```python
from build123d import *

# Parameters (mm, degrees)
SKETCH1_W           = 25.4
SKETCH1_H           = 25.4
BOSS_EXTRUDE1_DEPTH = 38.1
CUT_EXTRUDE1_DEPTH  = 43.121134838
CUT_EXTRUDE2_START  = -3.175
CUT_EXTRUDE2_DEPTH  = 31.75
SKETCH4_R           = 3.175
CUT_EXTRUDE3_DEPTH  = 48.519048812
SKETCH5_R           = 3.175
CUT_EXTRUDE5_DEPTH  = 48.519048812


with BuildPart() as part:
    # Sketch1 → Boss-Extrude1 (new body)
    with BuildSketch(Plane(origin=(0, 0, 0), x_dir=(1, 0, 0), z_dir=(0, 1, 0))):
        Rectangle(SKETCH1_W, SKETCH1_H)
    extrude(amount=BOSS_EXTRUDE1_DEPTH)

    # Sketch2 → Cut-Extrude1 (cut, through all)
    with BuildSketch(Plane(origin=(0, 38.1, 0), x_dir=(1, 0, 0), z_dir=(0, 1, 0))):
        Polygon((-12.7, 12.7), (12.7, -12.7), (-12.7, -12.7), align=None)
    extrude(amount=-CUT_EXTRUDE1_DEPTH, mode=Mode.SUBTRACT)

    # Sketch3 → Cut-Extrude2 (cut)
    with BuildSketch(Plane(origin=(0, 38.1, 0), x_dir=(1, 0, 0), z_dir=(0, 1, 0)).offset(CUT_EXTRUDE2_START)):
        Polygon((-9.525, 9.525), (9.525, 9.525), (9.525, -9.525), align=None)
    extrude(amount=-CUT_EXTRUDE2_DEPTH, mode=Mode.SUBTRACT)

    # Sketch4 → Cut-Extrude3 (cut, through all)
    with BuildSketch(Plane(origin=(0, 0, -12.7), x_dir=(-1, 0, 0), z_dir=(0, 0, -1))):
        with Locations((0, 19.05)):
            Circle(SKETCH4_R)
    extrude(amount=-CUT_EXTRUDE3_DEPTH, mode=Mode.SUBTRACT)

    # Sketch5 → Cut-Extrude5 (cut, through all)
    with BuildSketch(Plane(origin=(12.7, 0, 0), x_dir=(0, 0, -1), z_dir=(1, 0, 0))):
        with Locations((0, 31.75)):
            Circle(SKETCH5_R)
        with Locations((0, 6.35)):
            Circle(SKETCH5_R)
    extrude(amount=-CUT_EXTRUDE5_DEPTH, mode=Mode.SUBTRACT)


solid = part.part
```
CAD build for the part. Positions are in the model's coordinates, mm. A direction names the side the tool comes from. Coordinates: 2 decimals unless noted, no trailing zeros. Loops run counter-clockwise (first coordinate to the right, second up) from the corner with the lowest first, then second, coordinate; pieces in that order, holes last. Notation, with made-up numbers: (88, 57.5) - (101, 57.5) arc R22 ccw to (101, 79.5) - close; hole circle Ø7 at (35.5, 32.25). An arc over 180 degrees is marked (long way). Use CSV: the item, a comma, the result in double quotes. Start each with the question number.
Q1. Cut at C-C, the plane x = 5.25. List the corners of the cut face in (y, z) (3 decimals).
Q2. Cut at D-D, the plane y = 6.35. List the corners of the cut face in (x, z) (3 decimals), then the cut area to 3 significant figures.
Q3. Two-plate mould, pull along Y, no slides. Class faces 3 (the cylindrical face through (0.69, 15.95, -11.13)), 4 (the flat face through (5, 38.1, -6)), 5 (the flat face through (5, 0, -6)), 6 (the flat face through (0, 23, -12.7)): +Y half, -Y half, draft (parallel to the pull), parting line (faces both ways), or undercut.
Q4. Probe probe 1 along Y at (x, z) = (11.7, 0) (3 decimals); probe 2 along Y at (x, z) = (3.5, 0.75) (3 decimals); probe 3 along Y at (x, z) = (0, -11.95) (3 decimals). List the from-to ranges inside material, lowest first. Write a range as from..to.
Q5. 3-axis set-ups, long thin cutter, end or side, ignore diameter. For faces 1 (the cylindrical face through (11.135, 9.027, -1.707)), 2 (the flat face through (9.525, 19, 0)): which of +Z, -Z, +X, -X, +Y, -Y reach the whole face in a straight line?
Q6. Drop flat-ended pins along their axis: P1, Ø4, axis at y = 18, z = -1, coming from the -X side (3 decimals); P2, Ø1, axis at x = -4, y = 12.5, coming from the +Z side (3 decimals). Give the stop position or say it passes through.
Q7. Cut at B-B, the plane z = 8.75. List the corners of the cut face in (x, y) (3 decimals).
Q8. Cut at A-A, the plane y = 19.05. List the corners of the cut face in (x, z) (3 decimals), then the cut area to 3 significant figures.
Here are the results:
1,outline,"(0, -12.7) - (38.1, -12.7) - (38.1, 5.25) - (34.925, 5.25) - (34.925, -9.525) - (3.175, -9.525) - (3.175, 5.25) - (0, 5.25) - close"
2,outline,"(-12.7, -12.7) - (12.7, -12.7) - (12.7, -3.175) - (9.525, -3.175) - (9.525, -9.525) - (-9.525, -9.525) - close; (9.525, 3.175) - (12.7, 3.175) - (12.7, 12.7) - (9.525, 9.525) - close"
2,area,"121 mm2"
3,face 3,"undercut"
3,face 4,"+Y half"
3,face 5,"-Y half"
3,face 6,"draft"
4,probe 1,"0..3.175, 9.525..28.575, 34.925..38.1"
4,probe 2,"0..3.175, 34.925..38.1"
4,probe 3,"0..15.875, 22.225..38.1"
5,face 1,"+X, -X"
5,face 2,"+Z, -X"
6,P1,"x = 9.525"
6,P2,"z = -9.525"
7,outline,"(8.75, 0) - (12.7, 0) - (12.7, 38.1) - (8.75, 38.1) - (8.75, 34.925) - (9.525, 34.925) - (9.525, 3.175) - (8.75, 3.175) - close"
8,outline,"(-12.7, -12.7) - (-3.175, -12.7) - (-3.175, -9.525) - (-9.525, -9.525) - close; (3.175, -12.7) - (12.7, -12.7) - (12.7, 12.7) - (9.525, 9.525) - (9.525, -9.525) - (3.175, -9.525) - close"
8,area,"121 mm2"
